Design review of the part built by this model. Coordinates are the model's own, in mm. Give positions to 0.01 mm unless a question says otherwise; leave off trailing zeros. Loops run counter-clockwise (first coordinate to the right, second up) from the corner with the lowest first, then second, coordinate; pieces in that order, holes last. Notation, with made-up numbers: (10, 25.5) - (37, 25.5) arc R29 cw to (37, 48.5) - close; hole circle Ø4 at (89.5, 7). An arc over 180 degrees is marked (long way). One line per item, written item: value. Start each with the question number.
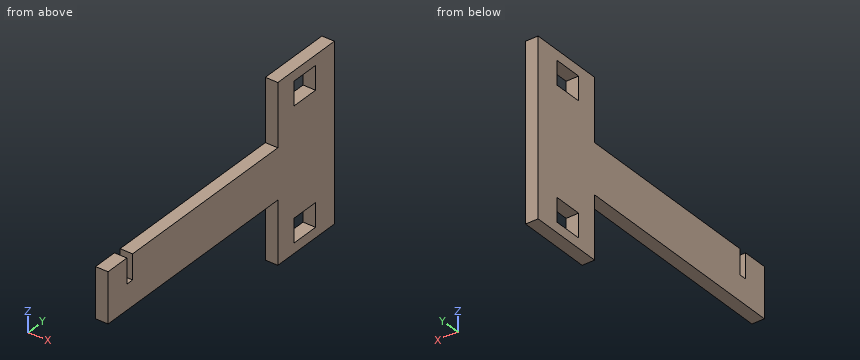
```python
from build123d import *

# Parameters (mm, degrees)
SKETCH1_W           = 5
SKETCH1_H           = 120
BOSS_EXTRUDE1_DEPTH = 70
SKETCH2_W           = 35
SKETCH2_H           = 3
CUT_EXTRUDE1_DEPTH  = 6
SKETCH3_W           = 9.5
SKETCH3_H           = 11.5
CUT_EXTRUDE2_DEPTH  = 6
SKETCH5_W           = 25
SKETCH5_H           = 90
CUT_EXTRUDE3_DEPTH  = 10


with BuildPart() as part:
    # Sketch1 → Boss-Extrude1 (new body)
    with BuildSketch(Plane.XY):
        with Locations((2.5, 60)):
            Rectangle(SKETCH1_W, SKETCH1_H)
    extrude(amount=BOSS_EXTRUDE1_DEPTH)

    # Sketch2 → Cut-Extrude1 (cut, through all)
    with BuildSketch(Plane(origin=(5, 0, 0), x_dir=(0, 0, -1), z_dir=(1, 0, 0))):
        with Locations((-52.5, 11.5)):
            Rectangle(SKETCH2_W, SKETCH2_H)
    extrude(amount=-CUT_EXTRUDE1_DEPTH, mode=Mode.SUBTRACT)

    # Sketch3 → Cut-Extrude2 (cut, through all)
    with BuildSketch(Plane(origin=(0, 0, 0), x_dir=(0, 0, -1), z_dir=(1, 0, 0))):
        with Locations((-8.75, 104.25)):
            Rectangle(SKETCH3_W, SKETCH3_H)
        with Locations((-61.25, 104.25)):
            Rectangle(SKETCH3_W, SKETCH3_H)
    extrude(amount=CUT_EXTRUDE2_DEPTH, mode=Mode.SUBTRACT)

    # Sketch5 → Cut-Extrude3 (cut)
    with BuildSketch(Plane(origin=(5, 0, 0), x_dir=(0, 0, -1), z_dir=(1, 0, 0))):
        with Locations((-57.5, 45)):
            Rectangle(SKETCH5_W, SKETCH5_H)
        with Locations((-12.5, 45)):
            Rectangle(SKETCH5_W, SKETCH5_H)
    extrude(amount=-CUT_EXTRUDE3_DEPTH, mode=Mode.SUBTRACT)


solid = part.part
```
(1) For pin 1 Ø2.5 at (x, y) = (2.5, 11) entering from +Z; pin 2 Ø2.5 at (x, z) = (3, 59.5) entering from -Y, all flat-tipped, find the tip position at first contact; note any pin that passes through.
(2) Take a section at A-A on x = 4. State the section outline as (y, z) points, and give its area (3 significant figures).
(3) Take a section at C-C on y = 66.5. State the section outline as (x, z) points, and give its area (3 significant figures).
(4) To check wall thickness, follow L1, parallel to Y at x = 4.7, z = 64; L2, parallel to Y at x = 0.25, z = 35.5; L3, parallel to Z at x = 1.65, y = 55.5. State the ranges of each line that lie inside material, in increasing order. Write a range as from..to.
(5) Take a section at B-B on z = 23.5. State the section outline as (x, y) points, and give its area (3 significant figures).
Here are the results:
1. pin 1: z = 45
1. pin 2: y = 90
2. outline: (0, 25) - (90, 25) - (90, 0) - (120, 0) - (120, 70) - (90, 70) - (90, 45) - (13, 45) - (13, 35) - (10, 35) - (10, 45) - (0, 45) - close; hole (98.5, 4) - (110, 4) - (110, 13.5) - (98.5, 13.5) - close; hole (98.5, 56.5) - (110, 56.5) - (110, 66) - (98.5, 66) - close
2. area: 3,650 mm²
3. outline: (0, 25) - (5, 25) - (5, 45) - (0, 45) - close
3. area: 100 mm²
4. L1: 90..98.5, 110..120
4. L2: 0..10, 13..120
4. L3: 25..45
5. outline: (0, 90) - (5, 90) - (5, 120) - (0, 120) - close
5. area: 150 mm²
